Could you check a few things on this model? Use its own coordinates, in mm. Give positions to 0.01 mm unless a question says otherwise; leave off trailing zeros. Loops run counter-clockwise (first coordinate to the right, second up) from the corner with the lowest first, then second, coordinate; pieces in that order, holes last. Notation, with made-up numbers: (-19.75, 5) - (-1.75, 5) arc R19 cw to (-1.75, 32) - close; hole circle Ø7 at (35.25, 56.5). An arc over 180 degrees is marked (long way). Write each question's results on one line, items separated by ' | '. Start each with the question number.
```python
from build123d import *

# Parameters (mm, degrees)
F2_W     = 0.7
F2_H     = 0.7
F3_DEPTH = 13
F4_DEPTH = 6


with BuildPart() as f1:
    # F0 (on Front) → F1 (revolve)
    with BuildSketch(Plane.XZ):
        Polygon((0, 2), (0, 0), (7.25, 0), (9.25, 1), (9.25, 9.5), (8.25, 9.5), (8.25, 2.5), (7, 2), align=None)
    revolve(axis=Axis((0, 0, -0.2857148442), (0, 0, -1)))

    # F2 (on Top) → F3 (join)
    with BuildSketch(Plane.XY):
        with BuildLine():
            Line((-2.9795133831, -0.35), (-3.6834087473, -0.35))
            ThreePointArc((-3.6834087473, -0.35), (-2.9989376836, -2.1671116191), (-1.4885221007, -3.3873739026))
            Line((-1.4885221007, -3.3873739026), (-1.4885221007, -4.1405678301))
            ThreePointArc((-1.4885221007, -4.1405678301), (-1.1424042215, -4.2491072703), (-0.7885221007, -4.3287680576))
            Line((-0.7885221007, -4.3287680576), (-0.7885221007, -3.6150010922))
            Line((-0.7885221007, -3.6150010922), (-0.7885221007, -2.8945177313))
            ThreePointArc((-0.7885221007, -2.8945177313), (-2.2733599524, -1.9575072227), (-2.9795133831, -0.35))
        make_face()
        with BuildLine():
            Line((-0.35, 1.85), (-0.35, 2.55))
            Line((-0.35, 2.55), (-2.6809513237, 2.55))
            ThreePointArc((-2.6809513237, 2.55), (-3.366937745, 1.5341871534), (-3.6834087473, 0.35))
            Line((-3.6834087473, 0.35), (-2.9795133831, 0.35))
            ThreePointArc((-2.9795133831, 0.35), (-2.7739084983, 1.1425548752), (-2.3616731357, 1.85))
            Line((-2.3616731357, 1.85), (-0.35, 1.85))
        make_face()
        with BuildLine():
            Line((2.6809513237, 2.55), (0.35, 2.55))
            Line((0.35, 2.55), (0.35, 1.85))
            Line((0.35, 1.85), (2.3616731357, 1.85))
            ThreePointArc((2.3616731357, 1.85), (2.7739084983, 1.1425548752), (2.9795133831, 0.35))
            Line((2.9795133831, 0.35), (3.6834087473, 0.35))
            ThreePointArc((3.6834087473, 0.35), (3.366937745, 1.5341871534), (2.6809513237, 2.55))
        make_face()
        with BuildLine():
            ThreePointArc((3.6834087473, -0.35), (3.7, 0), (3.6834087473, 0.35))
            Line((3.6834087473, 0.35), (2.9795133831, 0.35))
            ThreePointArc((2.9795133831, 0.35), (3, 0), (2.9795133831, -0.35))
            Line((2.9795133831, -0.35), (3.6834087473, -0.35))
        make_face()
        with Locations((0, 2.2)):
            Rectangle(F2_W, F2_H)
        with BuildLine():
            Line((-2.9795133831, 0.35), (-3.6834087473, 0.35))
            ThreePointArc((-3.6834087473, 0.35), (-3.7, 0), (-3.6834087473, -0.35))
            Line((-3.6834087473, -0.35), (-2.9795133831, -0.35))
            ThreePointArc((-2.9795133831, -0.35), (-3, 0), (-2.9795133831, 0.35))
        make_face()
        with BuildLine():
            ThreePointArc((1.4885221007, -3.3873739026), (2.9989376836, -2.1671116191), (3.6834087473, -0.35))
            Line((3.6834087473, -0.35), (2.9795133831, -0.35))
            ThreePointArc((2.9795133831, -0.35), (2.2733599524, -1.9575072227), (0.7885221007, -2.8945177313))
            Line((0.7885221007, -2.8945177313), (0.7885221007, -3.6150010922))
            Line((0.7885221007, -3.6150010922), (0.7885221007, -4.3287680576))
            ThreePointArc((0.7885221007, -4.3287680576), (1.1424042215, -4.2491072703), (1.4885221007, -4.1405678301))
            Line((1.4885221007, -4.1405678301), (1.4885221007, -3.3873739026))
        make_face()
        with BuildLine():
            ThreePointArc((-3.6834087473, -0.35), (-3.7, 0), (-3.6834087473, 0.35))
            Line((-3.6834087473, 0.35), (-4.3860574552, 0.35))
            ThreePointArc((-4.3860574552, 0.35), (-4.4, 0), (-4.3860574552, -0.35))
            Line((-4.3860574552, -0.35), (-3.6834087473, -0.35))
        make_face()
        with BuildLine():
            Line((0.35, 2.55), (0.35, 2.9795133831))
            ThreePointArc((0.35, 2.9795133831), (0, 3), (-0.35, 2.9795133831))
            Line((-0.35, 2.9795133831), (-0.35, 2.55))
            Line((-0.35, 2.55), (0.35, 2.55))
        make_face()
        with BuildLine():
            Line((4.3860574552, 0.35), (3.6834087473, 0.35))
            ThreePointArc((3.6834087473, 0.35), (3.7, 0), (3.6834087473, -0.35))
            Line((3.6834087473, -0.35), (4.3860574552, -0.35))
            ThreePointArc((4.3860574552, -0.35), (4.4, 0), (4.3860574552, 0.35))
        make_face()
    extrude(amount=F3_DEPTH)

    # F2 (on Top) → F4 (join)
    with BuildSketch(Plane.XY):
        with BuildLine():
            Line((0.35, 0.35), (0.35, 1.85))
            Line((0.35, 1.85), (-0.35, 1.85))
            Line((-0.35, 1.85), (-0.35, 0.35))
            Line((-0.35, 0.35), (-2.9795133831, 0.35))
            ThreePointArc((-2.9795133831, 0.35), (-3, 0), (-2.9795133831, -0.35))
            Line((-2.9795133831, -0.35), (-0.35, -0.35))
            Line((-0.35, -0.35), (-0.35, -2.9795133831))
            ThreePointArc((-0.35, -2.9795133831), (-0.5708451705, -2.9451885833), (-0.7885221007, -2.8945177313))
            Line((-0.7885221007, -2.8945177313), (-0.7885221007, -3.6150010922))
            ThreePointArc((-0.7885221007, -3.6150010922), (0, -3.7), (0.7885221007, -3.6150010922))
            Line((0.7885221007, -3.6150010922), (0.7885221007, -2.8945177313))
            ThreePointArc((0.7885221007, -2.8945177313), (0.5708451705, -2.9451885833), (0.35, -2.9795133831))
            Line((0.35, -2.9795133831), (0.35, -0.35))
            Line((0.35, -0.35), (2.9795133831, -0.35))
            ThreePointArc((2.9795133831, -0.35), (3, 0), (2.9795133831, 0.35))
            Line((2.9795133831, 0.35), (0.35, 0.35))
        make_face()
    extrude(amount=F4_DEPTH)


solid = f1.part
```
Q1. If we mould it in two halves opening along Y, with no side actions, what happens to faces 1 (the face through (-0.789, -4, 9)), 2 (the face through (-1, -1, 2)), 3 (the face through (0, 0, 0))? For each: +Y half, -Y half, draft (parallel to the pull), parting line (faces both ways), or undercut.
Q2. I want a section at D-D, the plane y = 0. List the corners of the cut face in (x, z) for me.
Q3. I want a section at A-A, the plane z = 9. List the corners of the cut face in (x, y) for me, then the cut area to 3 significant figures.
Q4. I need wall thicknesses on L1, parallel to Y at x = 0, z = 5.5; L2, parallel to Y at x = 0, z = 6.25; L3, parallel to Y at x = -1.25, z = 4. Which ranges of each line are inside material? Lowest first, please. Write a range as from..to.
Q5. I'm going to push flat-ended pins straight in: pin 1 Ø0.8 at (x, z) = (2.5, 4.5) entering from +Y; pin 2 Ø1 at (y, z) = (-4.5, 6) entering from -X; pin 3 Ø1.1 at (y, z) = (-3.5, 9) entering from +X. Where does each tip first touch, or does it pass through?
Q6. I want a section at B-B, the plane x = 0. List the corners of the cut face in (y, z) for me.
Q7. I want a section at C-C, the plane z = 2.75. State how many separate pieces and enclosed holes the cut face has, then the cut area to 3 significant figures.
Conclusion:
1) face 1: undercut | face 2: undercut | face 3: draft
2) outline: (-9.25, 1) - (-7.25, 0) - (7.25, 0) - (9.25, 1) - (9.25, 9.5) - (8.25, 9.5) - (8.25, 2.5) - (7, 2) - (4.4, 2) - (4.4, 13) - (3, 13) - (3, 6) - (-3, 6) - (-3, 13) - (-4.4, 13) - (-4.4, 2) - (-7, 2) - (-8.25, 2.5) - (-8.25, 9.5) - (-9.25, 9.5) - close
3) outline: circle Ø18.5 at (0, 0); (-4.39, -0.35) - (-3.68, -0.35) arc R3.7 ccw to (-1.49, -3.39) - (-1.49, -4.14) arc R4.4 ccw to (-0.79, -4.33) - (-0.79, -2.89) arc R3 cw to (-2.36, 1.85) - (2.36, 1.85) arc R3 cw to (0.79, -2.89) - (0.79, -4.33) arc R4.4 ccw to (1.49, -4.14) - (1.49, -3.39) arc R3.7 ccw to (3.68, -0.35) - (4.39, -0.35) arc R4.4 ccw to (4.39, 0.35) - (3.68, 0.35) arc R3.7 ccw to (2.68, 2.55) - (0.35, 2.55) - (0.35, 2.98) arc R3 ccw to (-0.35, 2.98) - (-0.35, 2.55) - (-2.68, 2.55) arc R3.7 ccw to (-3.68, 0.35) - (-4.39, 0.35) arc R4.4 ccw to start; hole circle Ø16.5 at (0, 0) | area: 70.4 mm^2
4) L1: -9.25..-8.25, -3.7..3, 8.25..9.25 | L2: -9.25..-8.25, 1.85..3, 8.25..9.25 | L3: -9.17..-8.15, -4.22..-2.73, -0.35..0.35, 1.85..2.55, 8.15..9.17
5) pin 1: y = 9.01 | pin 2: x = -8.34 | pin 3: x = 8.77
6) outline: (-9.25, 1) - (-7.25, 0) - (7.25, 0) - (9.25, 1) - (9.25, 9.5) - (8.25, 9.5) - (8.25, 2.5) - (7, 2) - (3, 2) - (3, 13) - (1.85, 13) - (1.85, 6) - (-3.7, 6) - (-3.7, 2) - (-7, 2) - (-8.25, 2.5) - (-8.25, 9.5) - (-9.25, 9.5) - close
7) separate pieces: 2 | enclosed holes: 5 | area: 78.6 mm^2
